Could you check a few things on this model? Use its own coordinates, in mm. Round coordinates to 2 decimals unless told otherwise and drop trailing zeros. Write each loop counter-clockwise with the first axis right and the second up, starting at its lowest first coordinate (ties: lowest second). Pieces come first, ordered by that corner, then holes. Notation, with made-up numbers: (-35.75, 6.25) -> (17.25, 6.25) arc R20 ccw to (17.25, 30.25) -> close; hole circle Ø9 at (7, 55). An arc over 180 degrees is marked (long way). One line per question, with ' | ' between items. Start each with the question number.
1. Imagine slicing it at A-A, the plane y = 7. List the corners of the cut face in (x, z) for me, and give its area (3 significant figures).
2. If I drill on line 1 along X through (y, z) = (20.5, 2.1); line 2 along X through (y, z) = (14.75, -2.1); line 3 along Z through (x, y) = (-15, 14.5), over which ranges is the centre line in solid material (lowest first)? Write a range as [from, to].
3. Thinking about a two-plate mould opening in X: for faces 1 (the cylindrical face through (-0.326, 12.115, 1.026)), 2 (the flat face through (-15, 27, -1)), 3 (the flat face through (-15, 13, 0)), which applies, released by +X, released by -X, zero draft, split by the parting line, or undercut?
4. For pin 1 Ø3 at (y, z) = (9.5, -1.5) entering from +X; pin 2 Ø2 at (y, z) = (5.5, 0) entering from +X, each with a flat end and sliding along its axis, tell me the tip position at first contact or that it passes through.
5. Imagine slicing it at B-B, the plane x = -8.5. List the corners of the cut face in (y, z) for me, and give its area (3 significant figures).
from build123d import *

# Parameters (mm, degrees)
BOSS_EXTRUDE1_DEPTH     = 27
CUT_EXTRUDE1_DEPTH      = 33.019431415
CUT_EXTRUDE1_DEPTH_BACK = 33.019431415
SKETCH2_R               = 14


with BuildPart() as part:
    # Sketch1 → Boss-Extrude1 (new body)
    with BuildSketch(Plane(origin=(0, 0, 0), x_dir=(1, 0, 0), z_dir=(0, 1, 0))):
        Polygon((-17.5, 2.5), (17.5, 2.5), (12.5, -2.5), (-12.5, -2.5), align=None)
    extrude(amount=BOSS_EXTRUDE1_DEPTH)

    # Sketch2 → Cut-Extrude1 (cut, two sides: drawn at the far end of the back side and taken through both)
    with BuildSketch(Plane(origin=(0, 0.625, 2.332531755), x_dir=(1, 0, 0), z_dir=(0, 0.25881904510251796, 0.9659258262890691)).offset(-CUT_EXTRUDE1_DEPTH_BACK)):
        with Locations((0, 25.432949697)):
            Circle(SKETCH2_R)
    extrude(amount=CUT_EXTRUDE1_DEPTH + CUT_EXTRUDE1_DEPTH_BACK, mode=Mode.SUBTRACT)


solid = part.part
Geometry results:
1) outline: (-17.5, -2.5) -> (17.5, -2.5) -> (12.5, 2.5) -> (-12.5, 2.5) -> close | area: 150 mm2
2) line 1: x = [-12.9, -12.56], [12.56, 12.9] | line 2: x = [-17.1, -9.1], [9.1, 17.1] | line 3: z = [-2.5, 0]
3) face 1: undercut | face 2: zero draft | face 3: released by -X
4) pin 1: stops at x = 17.5 | pin 2: stops at x = 16
5) outline: (0, -2.5) -> (14.14, -2.5) -> (15.48, 2.5) -> (0, 2.5) -> close | area: 74.1 mm2
